Autodesk Inventor part; units mm, degrees
ref_plane "Work Plane1" through (0, 0, 63.5) normal (0, 0, -1) x (-1, 0, 0)
ref_plane "YZ Plane" through (0, 0, 0) normal (1, 0, 0) x (0, 1, 0)
ref_plane "XZ Plane" through (0, 0, 0) normal (0, 1, 0) x (-1, 0, 0)
sketch "Sketch1" plane through (0, 0, 0) normal (0, 0, 1) x (1, 0, 0)
  line L0 (-85, -15) -> (85, -15)
  line L1 (85, -15) -> (85, 15)
  line L2 (85, 15) -> (-85, 15)
  line L3 (-85, 15) -> (-85, -15)
  line L4 (-85, -15) -> (85, 15) construction
  line L5 (85, -15) -> (-85, 15) construction
  circle A0 centre (-35, -40) radius 2.1
  circle A1 centre (80, -45) radius 2.1
  line L6 (85, -50) -> (75, -50)
  line L7 (75, -50) -> (75, -15) construction
  line L8 (75, -15) -> (85, -15)
  line L9 (85, -15) -> (85, -50)
  line L10 (85, -50) -> (75, -15) construction
  line L11 (75, -50) -> (85, -15) construction
  line L12 (-32.5, -15) -> (-47.5, -15)
  line L13 (-48, -15) -> (75, -15)
  line L14 (75, -45) -> (-48, -45)
  line L15 (-48, -45) -> (-48, -15)
  line L16 (-85, -5) -> (-48, -5)
  line L17 (-48, -5) -> (-48, -15)
  line L18 (85, -50) -> (80.4548, 15)
  line L19 (75, -50) -> (60, -45)
  point P0 (0, 0)
  point P1 (80, -32.5)
  point P2 (85, -15)
  point P3 (12.5, -15)
  point P4 (7.5, -15)
  point P5 (-47.5, -15)
  point P6 (-48, -15)
  point P7 (82.5526, -15)
  dimension "d0" = 170
  dimension "d1" = 30
  dimension "d2" = 4.2
  dimension "d5" = 4.2
  dimension "d7" = 5
  dimension "d10" = 30
  dimension "d14" = 13
  dimension "d15" = 30
  dimension "d18" = 25
  dimension "d19" = 35
  dimension "d20" = 20
  dimension "d21" = 37
  dimension "d36" = 4
  dimension "d43" = 15
extrude "Extrusion1" add sketch "Sketch1" along normal blind 127 contours L17 L16 L3 L2 L18 L0 | L0 L18 L6 L19 L14 L15 | A0 | A1
shell "Shell3" thickness 5 removed faces 2 at (83.4849, -28.3333, 42.3333) at (25.3032, 15, 42.3333)
extrude "Extrusion2" cut sketch "Sketch1" along normal blind 25 contours A0 | A1
sketch "Sketch2" plane through (0, 0, 127) normal (0, 0, 1) x (1, 0, 0)
  circle A0 centre (50, 5) radius 2.5
  line L0 (-85, 15) -> (-85, -5) construction
  line L1 (80.4548, 15) -> (-85, 15) construction
  line L2 (-48, -45) -> (60, -45)
  line L3 (60, -45) -> (75, -50)
  line L4 (75, -50) -> (85, -50)
  line L5 (85, -50) -> (80.4548, 15)
  line L6 (-85, -5) -> (-48, -5)
  line L7 (-48, -5) -> (-48, -45)
  point P0 (0, 0)
  dimension "d22" = 5
  dimension "d24" = 10
ref_plane "Work Plane1" through (0, 0, 63.5) normal (0, 0, -1) x (-1, 0, 0)
mirror "Mirror1" about plane through (0, 0, 63.5) normal (0, 0, -1) of "Extrusion2"
extrude "Extrusion4" cut sketch "Sketch2" against normal through all
chamfer "Chamfer2" distance 5 angle 45 2 edges at (80.4548, 15, 124.5) (80.4548, 15, 2.5)
sketch "Sketch3" plane through (0, 0, 127) normal (0, 0, 1) x (1, 0, 0)
  circle A0 centre (-35, -40) radius 2.1
  circle A1 centre (80, -45) radius 2.1
  point P0 (0, 0)
extrude "Extrusion5" cut sketch "Sketch3" against normal through all
equation "\"d5\" = d2"
properties part number "bed"
Check sheet for the modelled part. Datum: model origin and axes. Units: mm. A direction names the side the tool comes from. Coordinates: 2 decimals unless noted, no trailing zeros. Write each loop counter-clockwise with the first axis right and the second up, starting at its lowest first coordinate (ties: lowest second). Pieces come first, ordered by that corner, then holes. Notation, with made-up numbers: M 42.25,-9.5 L 97.25,-9.5 A32 cw 97.25,19.5 Z; hole C 39,72.25 d8. An arc over 180 degrees is marked long. Use one line per item in the form item = value.
Item 1: Release check for a two-part mould opening along X. For faces 4 (the face through (78.17, 12.47, 124.46)), 5 (the face through (19, -8, 122)), 6 (the face through (79.54, -47.05, 64.39)) record: pulls with the +X half, pulls with the -X half, needs draft (parallel to the pull), parting line crosses it, or undercut.
Answer below:
face_4 = pulls with the +X half
face_5 = needs draft
face_6 = undercut
Item 2: Sectioned sample at C-C, the plane x = 32. Record the cut outline in (y, z).
Answer below:
outline = M -45,0 L 15,0 L 15,5 L -40,5 L -40,122 L 15,122 L 15,127 L -45,127 Z
Item 3: Gauge pin test, flat ends, axial feed: pin 1 Ø1.5 at (y, z) = (-15, 41.5) entering from +X; pin 2 Ø3 at (x, z) = (84, 69) entering from +Y; pin 3 Ø12 at (y, z) = (-33.5, 52) entering from -X. Record the tip position at first contact, or that the pin passes through.
Answer below:
pin_1 = -43
pin_2 = -45
pin_3 = -48
Item 4: Sectioned sample at D-D, the plane y = 5. Record the cut outline in (x, z), and give its area (3 significant figures).
Answer below:
outline = M -85,0 L 47.5,0 L 47.5,5 L -80,5 L -80,122 L 47.5,122 L 47.5,127 L -85,127 Z; M 52.5,0 L 81.15,0 L 81.15,5 L 52.5,5 Z; M 52.5,122 L 81.15,122 L 81.15,127 L 52.5,127 Z
area = 2,200 mm^2
Item 5: Sectioned sample at A-A, the plane x = -35. Record the cut outline in (y, z), and give its area (3 significant figures).
Answer below:
outline = M -45,0 L -42.1,0 L -42.1,127 L -45,127 Z; M -37.9,0 L 15,0 L 15,5 L -37.9,5 Z; M -37.9,122 L 15,122 L 15,127 L -37.9,127 Z
area = 897 mm^2
Item 6: Material ranges on L1, parallel to Y at x = 50, z = 1.9; L2, parallel to Z at x = 1.5, y = -21.5; L3, parallel to Y at x = 80, z = 66, recorded low to high. Write a range as from..to.
Answer below:
L1 = -45..2.5, 7.5..15
L2 = 0..5, 122..127
L3 = -50..-47.1
Item 7: Sectioned sample at B-B, the plane z = 26. Record the cut outline in (x, y), and give its area (3 significant figures).
Answer below:
outline = M -85,-5 L -48,-5 L -48,-45 L 60,-45 L 75,-50 L 85,-50 L 84.65,-45 L 82.1,-45 A2.1 cw 77.9,-45 L 75.81,-45 L 60.81,-40 L -32.9,-40 A2.1 cw -37.1,-40 L -43,-40 L -43,0 L -80,0 L -80,15 L -85,15 Z
area = 1,110 mm^2
Item 8: Set-up check for faces 1 (the face through (68.416, -42.535, 62.681)), 2 (the face through (80, -50, 63)), 3 (the face through (7, -45, 63)): record each of +Z, -Z, +X, -X, +Y, -Y from which the full face is reachable in a straight line by a thin tool's end or side.
Answer below:
face_1 = +X, +Y
face_2 = +Z, -Z, +X, -X, -Y
face_3 = +Z, -Z, -X, -Y
